```python
from build123d import *

# Parameters (mm, degrees)
SKETCH1_W           = 100
SKETCH1_H           = 10
BOSS_EXTRUDE1_DEPTH = 10
SKETCH6_W           = 3
SKETCH6_H           = 10
BOSS_EXTRUDE2_DEPTH = 17
SKETCH8_W           = 2
SKETCH8_H           = 10
BOSS_EXTRUDE3_DEPTH = 5
BOSS_EXTRUDE4_DEPTH = 20
SKETCH2_W           = 10
SKETCH2_H           = 5
CUT_EXTRUDE1_DEPTH  = 10
CUT_EXTRUDE2_REACH  = 62.075
SKETCH10_R          = 2
SKETCH13_R          = 4
SKETCH13_R_2        = 1
CUT_EXTRUDE3_DEPTH  = 59.429444632
FILLET1_R           = 3
FILLET2_R           = 3
SKETCH14_W          = 5
SKETCH14_H          = 10
BOSS_EXTRUDE5_DEPTH = 5


with BuildPart() as part:
    # Sketch1 → Boss-Extrude1 (new body)
    with BuildSketch(Plane.XY):
        Rectangle(SKETCH1_W, SKETCH1_H)
    extrude(amount=BOSS_EXTRUDE1_DEPTH)

    # Sketch6 → Boss-Extrude2 (add)
    with BuildSketch(Plane(origin=(0, 0, 0), x_dir=(-1, 0, 0), z_dir=(0, 0, -1))):
        with Locations((-23.5, 0)):
            Rectangle(SKETCH6_W, SKETCH6_H)
    boss_extrude2 = extrude(amount=BOSS_EXTRUDE2_DEPTH)

    # Sketch8 → Boss-Extrude3 (add)
    with BuildSketch(Plane.ZY.offset(-22)):
        with Locations((-16, 0)):
            Rectangle(SKETCH8_W, SKETCH8_H)
    boss_extrude3 = extrude(amount=BOSS_EXTRUDE3_DEPTH)

    # Sketch9 → Boss-Extrude4 (add)
    with BuildSketch(Plane.XZ.offset(5)):
        Polygon((17, 2), (17, 0), (22, 0), (22, -15), (17, -15), (17, -17), (25, -17), (25, 0), (25, 2), align=None)
    boss_extrude4 = extrude(amount=BOSS_EXTRUDE4_DEPTH)

    # Mirror3: Boss-Extrude2, Boss-Extrude3, Boss-Extrude4 across plane
    add(boss_extrude2.mirror(Plane(origin=(0, 0, 0), x_dir=(0, 0, 1), z_dir=(1, 0, 0))))
    add(boss_extrude3.mirror(Plane(origin=(0, 0, 0), x_dir=(0, 0, 1), z_dir=(1, 0, 0))))
    add(boss_extrude4.mirror(Plane(origin=(0, 0, 0), x_dir=(0, 0, 1), z_dir=(1, 0, 0))))

    # Sketch2 → Cut-Extrude1 (cut)
    with BuildSketch(Plane(origin=(0, 5, 0), x_dir=(1, 0, 0), z_dir=(0, 1, 0))):
        with Locations((-45, -7.5)):
            Rectangle(SKETCH2_W, SKETCH2_H)
    cut_extrude1 = extrude(amount=-CUT_EXTRUDE1_DEPTH, mode=Mode.SUBTRACT)

    # Mirror4: Cut-Extrude1 across plane
    add(cut_extrude1.mirror(Plane(origin=(0, 0, 0), x_dir=(0, 0, 1), z_dir=(1, 0, 0))), mode=Mode.SUBTRACT)

    # Sketch10 → Cut-Extrude2 (cut, up to next)
    with BuildSketch(Plane.XY.offset(5), mode=Mode.PRIVATE) as cut_extrude2_sk1:
        with Locations((45, 0)):
            Circle(SKETCH10_R)
    cut_extrude2_tool1 = extrude(cut_extrude2_sk1.sketch, amount=-CUT_EXTRUDE2_REACH, mode=Mode.PRIVATE) & part.part
    cut_extrude2 = cut_extrude2_tool1.solids().sort_by_distance((45, 0, 5))[0]
    add(cut_extrude2, mode=Mode.SUBTRACT)

    # Mirror5: Cut-Extrude2 across plane
    add(cut_extrude2.mirror(Plane(origin=(0, 0, 0), x_dir=(0, 0, 1), z_dir=(1, 0, 0))), mode=Mode.SUBTRACT)

    # Sketch13 → Cut-Extrude3 (cut, through all)
    with BuildSketch(Plane(origin=(0, 0, 0), x_dir=(-1, 0, 0), z_dir=(0, 0, -1))):
        Circle(SKETCH13_R)
        with Locations((-8.5, 0)):
            Circle(SKETCH13_R_2)
        with Locations((8.5, 0)):
            Circle(SKETCH13_R_2)
    extrude(amount=-CUT_EXTRUDE3_DEPTH, mode=Mode.SUBTRACT)

    # Fillet1
    fillet1_edges = [part.edges().sort_by_distance(p)[0] for p in [
        (25, -10, -17),
        (-25, -10, -17),
    ]]
    fillet(fillet1_edges, radius=FILLET1_R)

    # Fillet2
    fillet2_edges = [part.edges().sort_by_distance(p)[0] for p in [
        (-25, -15, 2),
        (25, -15, 2),
    ]]
    fillet(fillet2_edges, radius=FILLET2_R)

    # Sketch14 → Boss-Extrude5 (add)
    with BuildSketch(Plane(origin=(0, 0, 0), x_dir=(-1, 0, 0), z_dir=(0, 0, -1))):
        with Locations((19.5, 0)):
            Rectangle(SKETCH14_W, SKETCH14_H)
    boss_extrude5 = extrude(amount=BOSS_EXTRUDE5_DEPTH)

    # Mirror6: Boss-Extrude5 across plane
    add(boss_extrude5.mirror(Plane(origin=(0, 0, 0), x_dir=(0, 0, 1), z_dir=(1, 0, 0))))


solid = part.part
```
CAD build for the part. Positions are in the model's coordinates, mm. A direction names the side the tool comes from. Give positions to 0.01 mm unless a question says otherwise; leave off trailing zeros. Loops run counter-clockwise (first coordinate to the right, second up) from the corner with the lowest first, then second, coordinate; pieces in that order, holes last. Notation, with made-up numbers: (-20.5, 84.5) -> (21.5, 84.5) arc R30 ccw to (21.5, 119.5) -> close; hole circle Ø1 at (14, 34.25). An arc over 180 degrees is marked (long way). Use a Markdown table: item, result.
1. Slice it at C-C (y = -9.5). List the corners of the cut face in (x, z), plus the area to 3 significant figures.
Check result:
| item | result |
|---|---|
| outline | (-25, -14) arc R3 ccw to (-22, -17) -> (-17, -17) -> (-17, -15) -> (-22, -15) -> (-22, 0) -> (-17, 0) -> (-17, 2) -> (-22, 2) arc R3 ccw to (-25, -1) -> close; (17, -17) -> (22, -17) arc R3 ccw to (25, -14) -> (25, -1) arc R3 ccw to (22, 2) -> (17, 2) -> (17, 0) -> (22, 0) -> (22, -15) -> (17, -15) -> close |
| area | 146 mm^2 |
2. Mould opens along X. For faces 1 (the flat face through (-40, 0, 8)), 2 (the cylindrical face through (0.867, -3.905, 4.93)), 3 (the flat face through (-1, 5, 3)), 4 (the flat face through (17, 0, -2)) say: pulls with the +X half, pulls with the -X half, needs draft (parallel to the pull), parting line crosses it, or undercut.
Check result:
| item | result |
|---|---|
| face 1 | pulls with the -X half |
| face 2 | undercut |
| face 3 | needs draft |
| face 4 | undercut |
3. Wall check: L1, parallel to X at y = -15.25, z = -2; L2, parallel to Y at x = 0, z = 6.25; L3, parallel to X at y = 1.25, z = -2.25. Give the ranges that are in metal, low to high. Write a range as [from, to].
Check result:
| item | result |
|---|---|
| L1 | x = [-25, -22], [22, 25] |
| L2 | y = [-5, -4], [4, 5] |
| L3 | x = [-25, -17], [17, 25] |
4. Slice it at B-B (x = 19.5). List the corners of the cut face in (y, z).
Check result:
| item | result |
|---|---|
| outline | (-25, -17) -> (5, -17) -> (5, -15) -> (-25, -15) -> close; (-25, 0) -> (-5, 0) -> (-5, -5) -> (5, -5) -> (5, 10) -> (-5, 10) -> (-5, 2) -> (-25, 2) -> close |
5. Slice it at D-D (z = -7). List the corners of the cut face in (x, y), plus the area to 3 significant figures.
Check result:
| item | result |
|---|---|
| outline | (-25, -25) -> (-22, -25) -> (-22, 5) -> (-25, 5) -> close; (22, -25) -> (25, -25) -> (25, 5) -> (22, 5) -> close |
| area | 180 mm^2 |
6. Slice it at A-A (z = -2.75). List the corners of the cut face in (x, y).
Check result:
| item | result |
|---|---|
| outline | (-25, -25) -> (-22, -25) -> (-22, -5) -> (-17, -5) -> (-17, 5) -> (-25, 5) -> close; (17, -5) -> (22, -5) -> (22, -25) -> (25, -25) -> (25, 5) -> (17, 5) -> close |
7. Flat gauge pins, fed straight in: pin 1 (1.6 mm diameter, centred on y = -16, z = 1, fed in from -X); pin 2 (1.5 mm diameter, centred on x = 29.5, y = -7, fed in from -Z); pin 3 (8 mm diameter, centred on x = 46.5, y = 1, fed in from +Z); pin 4 (5.5 mm diameter, centred on x = -18.5, y = -9, fed in from +Z). Where does each tip first touch, or does it go through?
Check result:
| item | result |
|---|---|
| pin 1 | stops at x = -24.75 |
| pin 2 | passes through |
| pin 3 | stops at z = 5 |
| pin 4 | stops at z = 2 |
8. Which spindle directions (+Z, -Z, +X, -X, +Y, -Y) get a long thin tool onto all of the face, cutting with end or side? Do faces 5 (the flat face through (-38, 0, 0)), 6 (the flat face through (-17, -10, -16)), 7 (the flat face through (-19, -5, -2)). Say none if no direction does.
Check result:
| item | result |
|---|---|
| face 5 | -Z, -X, +Y, -Y |
| face 6 | -Z, +Y, -Y |
| face 7 | -Y |
